Geometry check sheet. Reference: the model listing, model coordinates, mm. A direction names the side the tool comes from. Round coordinates to 2 decimals unless told otherwise and drop trailing zeros. Loops run counter-clockwise (first coordinate to the right, second up) from the corner with the lowest first, then second, coordinate; pieces in that order, holes last.
```python
from build123d import *

# Parameters (mm, degrees)
BOSS_EXTRUDE1_DEPTH = 50
SKETCH2_W           = 50
SKETCH2_H           = 4
BOSS_EXTRUDE2_DEPTH = 10
SKETCH4_W           = 14
SKETCH4_H           = 36
BOSS_EXTRUDE3_DEPTH = 16
SKETCH5_W           = 14
SKETCH5_H           = 7
BOSS_EXTRUDE4_DEPTH = 4
SKETCH7_W           = 10
SKETCH7_H           = 10
BOSS_EXTRUDE5_DEPTH = 11
SKETCH8_R           = 0.4
CUT_EXTRUDE2_DEPTH  = 7


with BuildPart() as part:
    # Sketch1 → Boss-Extrude1 (new body)
    with BuildSketch(Plane.XY):
        Polygon((0, 0), (2, 0), (2, 3), (3, 3), (3, -1), (-1, -1), (-1, 3), (0, 3), align=None)
    extrude(amount=BOSS_EXTRUDE1_DEPTH)

    # Sketch2 → Boss-Extrude2 (add)
    with BuildSketch(Plane(origin=(3, 0, 0), x_dir=(0, 0, -1), z_dir=(1, 0, 0))):
        with Locations((-25, 1)):
            Rectangle(SKETCH2_W, SKETCH2_H)
    extrude(amount=BOSS_EXTRUDE2_DEPTH)

    # Sketch4 → Boss-Extrude3 (add)
    with BuildSketch(Plane.XZ.offset(1)):
        with Locations((6, 32)):
            Rectangle(SKETCH4_W, SKETCH4_H)
    extrude(amount=BOSS_EXTRUDE3_DEPTH)

    # Sketch5 → Boss-Extrude4 (add)
    with BuildSketch(Plane(origin=(0, 0, 14), x_dir=(-1, 0, 0), z_dir=(0, 0, -1))):
        with Locations((-6, -13.5)):
            Rectangle(SKETCH5_W, SKETCH5_H)
    extrude(amount=BOSS_EXTRUDE4_DEPTH)

    # Sketch7 → Boss-Extrude5 (add)
    with BuildSketch(Plane(origin=(13, 0, 0), x_dir=(0, 0, -1), z_dir=(1, 0, 0))):
        with Locations((-15.4, 8)):
            Rectangle(SKETCH7_W, SKETCH7_H)
    extrude(amount=-BOSS_EXTRUDE5_DEPTH)

    # Sketch8 → Cut-Extrude2 (cut)
    with BuildSketch(Plane.ZY.offset(-2)):
        with Locations((15.4, 10.1)):
            Circle(SKETCH8_R)
    extrude(amount=-CUT_EXTRUDE2_DEPTH, mode=Mode.SUBTRACT)


solid = part.part
```
1) Gauge pin test, flat ends, axial feed: pin 1 (3 mm diameter, centred on x = 10, z = 4.5, fed in from +Y); pin 2 (0.9 mm diameter, centred on y = 10, z = 15.5, fed in from -X); pin 3 (7.5 mm diameter, centred on x = 2.5, y = -13.5, fed in from -Z). Record the tip position at first contact, or that the pin passes through.
Report:
pin 1: stops at y = 3
pin 2: stops at x = 2
pin 3: stops at z = 10
2) Sectioned sample at A-A, the plane x = 5. Record the cut outline in (y, z), then the cut area to 4 significant figures.
Report:
outline: (-17, 10) - (-10, 10) - (-10, 14) - (-1, 14) - (-1, 0) - (3, 0) - (3, 10.4) - (13, 10.4) - (13, 20.4) - (3, 20.4) - (3, 50) - (-17, 50) - close; hole circle Ø0.8 at (10.1, 15.4)
area: 903.5 mm2
3) Sectioned sample at C-C, the plane x = 11. Record the cut outline in (y, z), then the cut area to 3 significant figures.
Report:
outline: (-17, 10) - (-10, 10) - (-10, 14) - (-1, 14) - (-1, 0) - (3, 0) - (3, 10.4) - (13, 10.4) - (13, 20.4) - (3, 20.4) - (3, 50) - (-17, 50) - close
area: 904 mm2
4) Mould release check, pull along Y, two halves, no side actions. Record for faces 1 (the face through (7, 3, 5)), 2 (the face through (13, -6, 31)), 3 (the face through (6, -10, 12)), 4 (the face through (6, -5, 14)): +Y half, -Y half, draft (parallel to the pull), parting line (faces both ways), or undercut.
Report:
face 1: +Y half
face 2: draft
face 3: undercut
face 4: undercut
5) Access from +Z, -Z, +X, -X, +Y, -Y to the whole of each face (thin tool, end or side, straight path). Record for faces 5 (the face through (6, -1, 7)), 6 (the face through (-0.5, 3, 24.6)), 7 (the face through (2, 4, 19)), 8 (the face through (8, 8, 20.4)), 9 (the face through (8, 8, 10.4)).
Report:
face 5: -Z, +X, -X
face 6: +Z, -Z, -X, +Y
face 7: +Z, -Z, +Y
face 8: +Z, +X, -X, +Y
face 9: -Z, +X, -X, +Y
6) Sectioned sample at D-D, the plane z = 5. Record the cut outline in (x, y), then the cut area to 3 significant figures.
Report:
outline: (-1, -1) - (13, -1) - (13, 3) - (2, 3) - (2, 0) - (0, 0) - (0, 3) - (-1, 3) - close
area: 50.0 mm2
7) Sectioned sample at B-B, the plane z = 42. Record the cut outline in (x, y), then the cut area to 3 significant figures.
Report:
outline: (-1, -17) - (13, -17) - (13, 3) - (2, 3) - (2, 0) - (0, 0) - (0, 3) - (-1, 3) - close
area: 274 mm2
8) Scan lines: line 1 along Y through (x, z) = (7.25, 15.4); line 2 along X through (y, z) = (2.25, 24); line 3 along Y through (x, z) = (6.25, 4.5). Record each from-to range of solid material in increasing order.
Report:
line 1: y = -17 to 9.7, 10.5 to 13
line 2: x = -1 to 0, 2 to 13
line 3: y = -1 to 3
